The listing builds one solid part. Answer for the finished solid, in the listing's coordinates (mm). Face numbers are marked on the shaded views. A direction names the side the tool comes from. Coordinates: 2 decimals unless noted, no trailing zeros. Loops run counter-clockwise (first coordinate to the right, second up) from the corner with the lowest first, then second, coordinate; pieces in that order, holes last. Notation, with made-up numbers: (10.25, 73.5) - (34.25, 73.5) arc R23 cw to (34.25, 104.5) - close; hole circle Ø4 at (49.5, 72). An arc over 180 degrees is marked (long way). One line per question, with ' | ' between items.
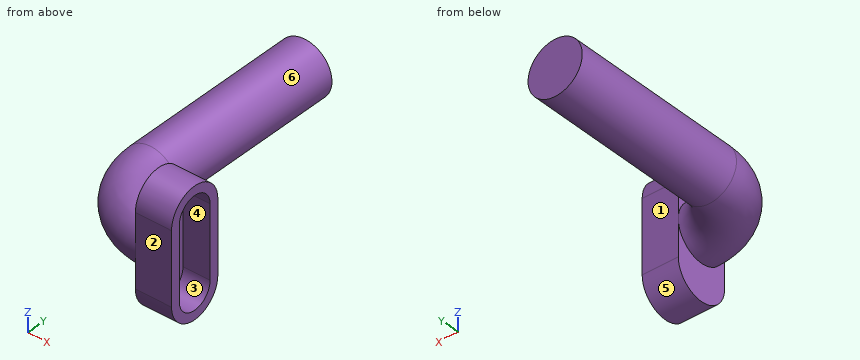
from build123d import *

# Parameters (mm, degrees)
BOSS_EXTRUDE1_DEPTH = 25.4
SHELL1_T            = -6.35
SKETCH7_R           = 19.05


with BuildPart() as part:
    # Sketch1 → Boss-Extrude1 (new body)
    with BuildSketch(Plane(origin=(0, 0, 0), x_dir=(0, 0, -1), z_dir=(1, 0, 0))):
        with BuildLine():
            Line((-25.4, 19.05), (25.4, 19.05))
            ThreePointArc((25.4, 19.05), (44.45, 0), (25.4, -19.05))
            Line((25.4, -19.05), (-25.4, -19.05))
            ThreePointArc((-25.4, -19.05), (-44.45, 0), (-25.4, 19.05))
        make_face()
    extrude(amount=BOSS_EXTRUDE1_DEPTH)

    # Shell1
    shell1_openings = [part.faces().sort_by_distance(p)[0] for p in [
        (25.4, 0, 0),
    ]]
    offset(amount=SHELL1_T, openings=shell1_openings, kind=Kind.INTERSECTION)

    # Sweep1: sweep along a path in Sketch3
    with BuildLine(Plane.XY) as sweep1_path:
        Line((-38.1, 165.1), (-38.1, 38.1))
        ThreePointArc((-38.1, 38.1), (-26.940768363, 11.159231637), (0, 0))
    # Sketch7 → Sweep1 (sweep)
    with BuildSketch(Plane.ZY):
        Circle(SKETCH7_R)
    sweep(path=sweep1_path.line)


solid = part.part
Item 1: Which of the six approach directions +Z, -Z, +X, -X, +Y, -Y give full straight-line access (tool end or side, diameter ignored) to the marked faces 1, 2 and 3?
Taken from the geometry:
face 1: +Z, -Z, +X, +Y | face 2: +Z, -Z, +X, -X, -Y | face 3: +X
Item 2: Find section A-A, the plane x = 14. Write down the section's boundary in (y, z), plus the area to 3 significant figures.
Taken from the geometry:
outline: (-19.05, -25.4) arc R19.05 ccw to (19.05, -25.4) - (19.05, 25.4) arc R19.05 ccw to (-19.05, 25.4) - close; hole (-12.7, -25.4) arc R12.7 ccw to (12.7, -25.4) - (12.7, 25.4) arc R12.7 ccw to (-12.7, 25.4) - close | area: 1,280 mm2
Item 3: Each of these flat-tipped pins is pushed along its axis until it touches: pin 1 Ø7.5 at (x, z) = (13, -3) entering from +Y; pin 2 Ø12 at (y, z) = (35, 10.5) entering from -X; pin 3 Ø1.5 at (y, z) = (33.5, -16.5) entering from +X. Where does it stop, or does it pass through?
Taken from the geometry:
pin 1: stops at y = 19.05 | pin 2: stops at x = -56.55 | pin 3: stops at x = -26.99
Item 4: Find section B-B, the plane z = 23.5. Write down the section's boundary in (x, y), plus the area to 3 significant figures.
Taken from the geometry:
outline: (0, -19.05) - (25.4, -19.05) - (25.4, -12.7) - (6.35, -12.7) - (6.35, 12.7) - (25.4, 12.7) - (25.4, 19.05) - (0, 19.05) - close | area: 484 mm2
Item 5: Find section C-C, the plane y = 67.5. Write down the section's boundary in (x, z).
Taken from the geometry:
outline: circle Ø38.1 at (-38.1, 0)
Item 6: Find section D-D, the plane z = -6.5. Write down the section's boundary in (x, y), plus the area to 3 significant figures.
Taken from the geometry:
outline: (-56.01, 38.1) arc R56.01 ccw to (0, -17.91) - (0, -19.05) - (25.4, -19.05) - (25.4, -12.7) - (6.35, -12.7) - (6.35, 12.7) - (25.4, 12.7) - (25.4, 19.05) - (0, 19.05) - (0, 17.91) arc R20.19 cw to (-20.19, 38.1) - (-20.19, 165.1) - (-56.01, 165.1) - close | area: 7,180 mm2
Item 7: The mould has two halves that part along Y. Classify the marked faces 4, 5 and 6: pulls with the +Y half, pulls with the -Y half, needs draft (parallel to the pull), parting line crosses it, or undercut.
Taken from the geometry:
face 4: undercut | face 5: parting line crosses it | face 6: needs draft
Item 8: Find the intervals of material crossed by line 1 (Y direction, x = 13, z = 11.5); line 2 (X direction, y = 8, z = 25); line 3 (Y direction, x = 8, z = 29.5), in increasing order. Write a range as [from, to].
Taken from the geometry:
line 1: y = [-19.05, -12.7], [12.7, 19.05] | line 2: x = [0, 6.35] | line 3: y = [-18.6, -12.02], [12.02, 18.6]
